Geometry check sheet. Reference: the model listing, model coordinates, mm. Round coordinates to 2 decimals unless told otherwise and drop trailing zeros. Write each loop counter-clockwise with the first axis right and the second up, starting at its lowest first coordinate (ties: lowest second). Pieces come first, ordered by that corner, then holes. Notation, with made-up numbers: (69, 19) -> (104, 19) arc R35 cw to (104, 51) -> close; hole circle Ø6 at (19, 69.5). An arc over 180 degrees is marked (long way). Put each result on its own line as item: value. Start each with the question number.
from build123d import *

# Parameters (mm, degrees)
SKETCH1_W           = 400
SKETCH1_H           = 452
BOSS_EXTRUDE1_DEPTH = 3
SKETCH4_R           = 16
CUT_EXTRUDE2_DEPTH  = 10
SKETCH5_W           = 400
SKETCH5_H           = 8
CUT_EXTRUDE3_DEPTH  = 4


with BuildPart() as part:
    # Sketch1 → Boss-Extrude1 (new body)
    with BuildSketch(Plane.XY):
        with Locations((200, 226)):
            Rectangle(SKETCH1_W, SKETCH1_H)
    extrude(amount=BOSS_EXTRUDE1_DEPTH)

    # Sketch4 → Cut-Extrude2 (cut)
    with BuildSketch(Plane.XY.offset(3)):
        with Locations((25, 35)):
            Circle(SKETCH4_R)
    extrude(amount=-CUT_EXTRUDE2_DEPTH, mode=Mode.SUBTRACT)

    # Sketch5 → Cut-Extrude3 (cut, through all)
    with BuildSketch(Plane(origin=(0, 0, 0), x_dir=(-1, 0, 0), z_dir=(0, 0, -1))):
        with Locations((-200, 448)):
            Rectangle(SKETCH5_W, SKETCH5_H)
    extrude(amount=-CUT_EXTRUDE3_DEPTH, mode=Mode.SUBTRACT)


solid = part.part
(1) Sectioned sample at B-B (y = 35). Record the cut outline in (x, z), and give its area (3 significant figures).
(2) Material ranges on L1, parallel to Y at x = 25, z = 1.65; L2, parallel to Y at x = 19, z = 2.4, recorded low to high. Write a range as from..to.
(3) Go/stop test with a flat-tipped pin: pin 1 Ø8 at (x, y) = (59, 355) entering from -Z. Record where the tip stops, or that it passes through.
(4) Mould release check, pull along Y, two halves, no side actions. Record for faces 1 (the cylindrical face through (21.53, 19.38, 1.52)), 2 (the flat face through (197, 225, 0)): +Y half, -Y half, draft (parallel to the pull), parting line (faces both ways), or undercut.
(5) Sectioned sample at A-A (x = 25). Record the cut outline in (y, z).
Found:
1. outline: (0, 0) -> (9, 0) -> (9, 3) -> (0, 3) -> close; (41, 0) -> (400, 0) -> (400, 3) -> (41, 3) -> close
1. area: 1,100 mm2
2. L1: 0..19, 51..444
2. L2: 0..20.17, 49.83..444
3. pin 1: z = 0
4. face 1: undercut
4. face 2: draft
5. outline: (0, 0) -> (19, 0) -> (19, 3) -> (0, 3) -> close; (51, 0) -> (444, 0) -> (444, 3) -> (51, 3) -> close
